Part print with two shaded views. Sizes in mm from the minimum x, y, z corner. A direction names the side the tool comes from. Round coordinates to 2 decimals unless told otherwise and drop trailing zeros. Order: outer loops, then holes, each group sorted by start corner. A loop starts at its lowest first (then second) coordinate and runs counter-clockwise, first axis right, second up. Notation, with made-up numbers: (7.5, 40.25) -> (52.5, 40.25) arc R23 ccw to (52.5, 57.25) -> close; hole circle Ø10 at (51, 1). An arc over 180 degrees is marked (long way). Put each result on its own line as item: value. Start each with the question number.
Q1. Cut at D-D, the plane y = 12.5. List the corners of the cut face in (x, z).
Q2. Cut at A-A, the plane z = 6.25. List the corners of the cut face in (x, y).
Q3. Cut at B-B, the plane z = 26.5. List the corners of the cut face in (x, y).
Q4. Probe L1, parallel to Z at x = 36, y = 7.25; L2, parallel to Y at x = 35, z = 6; L3, parallel to X at y = 1, z = 57. List the from-to ranges inside material, lowest first.
Q5. Flat gauge pins, fed straight in: P1, Ø3, axis at y = 8, z = 12.5, coming from the +X side; P2, Ø2, axis at y = 5.5, z = 30.5, coming from the -X side; P3, Ø4, axis at x = 19.5, y = 12.5, coming from the -Z side; P4, Ø4.5, axis at y = 7.5, z = 6.25, coming from the +X side. Where does each tip first touch, or does it go through?
Q6. Cut at C-C, the plane x = 66. List the corners of the cut face in (y, z).
Q7. 3-axis set-ups, long thin cutter, end or side, ignore diameter. For the marked faces 1, 2 and 3: which of +Z, -Z, +X, -X, +Y, -Y reach the whole face in a straight line?
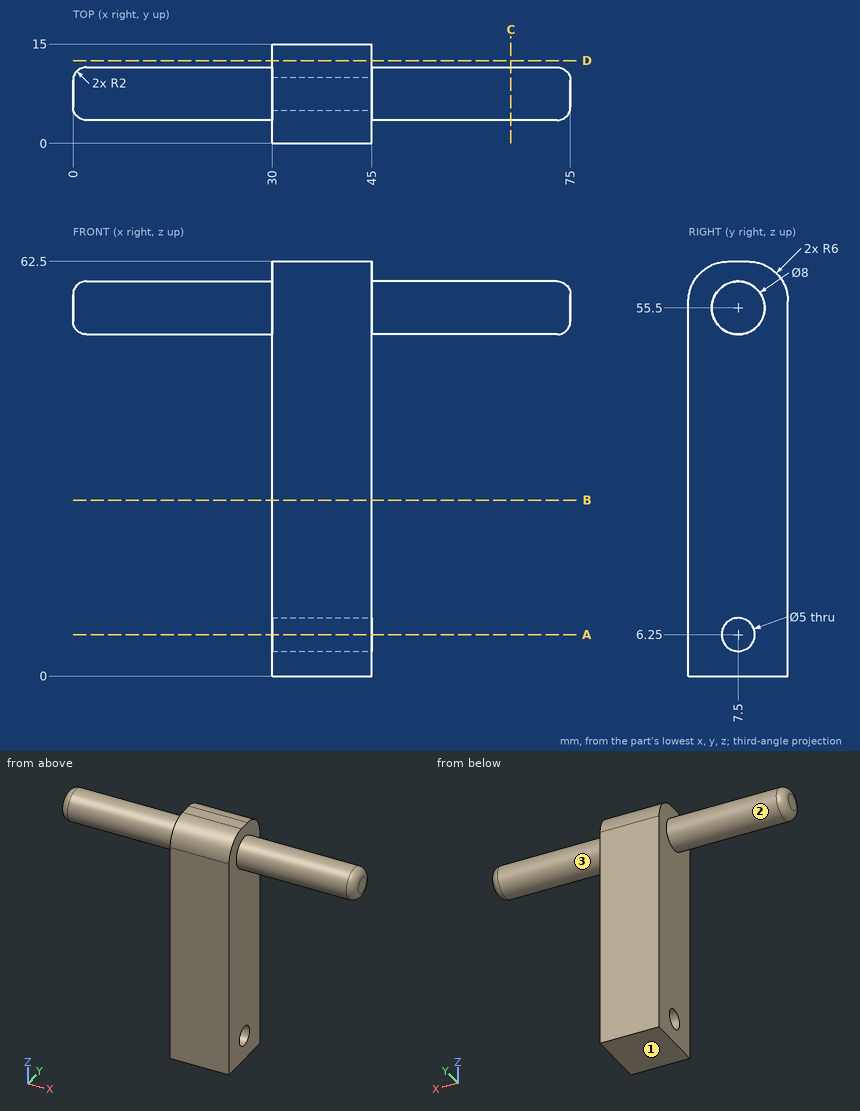
Ans:
1. outline: (30, 0) -> (45, 0) -> (45, 61.37) -> (30, 61.37) -> close
2. outline: (30, 0) -> (45, 0) -> (45, 5) -> (30, 5) -> close; (30, 10) -> (45, 10) -> (45, 15) -> (30, 15) -> close
3. outline: (30, 0) -> (45, 0) -> (45, 15) -> (30, 15) -> close
4. L1: z = 0 to 3.76, 8.74 to 62.5
4. L2: y = 0 to 5.01, 9.99 to 15
4. L3: x = 30 to 45
5. P1: stops at x = 45
5. P2: stops at x = 30
5. P3: stops at z = 52.85
5. P4: passes through
6. outline: circle Ø8 at (7.5, 55.5)
7. face 1: -Z, +X, -X, +Y, -Y
7. face 2: -X
7. face 3: +X
